from build123d import *

# Parameters (mm, degrees)
F0_R     = 60.325
F0_R_2   = 1.5875
F1_DEPTH = 3.175


with BuildPart() as f1:
    # F0 (on Front) → F1 (new body)
    with BuildSketch(Plane.XZ):
        Circle(F0_R)
        with BuildLine():
            ThreePointArc((-18.181951, -44.017693), (-39.585705, -26.478531), (-47.625, 0))
            Line((-47.625, 0), (-8.89, 0))
            ThreePointArc((-8.89, 0), (-7.82019, -4.228088), (-4.868239, -7.438571))
            Line((-4.868239, -7.438571), (-18.181951, -44.017693))
        make_face(mode=Mode.SUBTRACT)
        with BuildLine():
            ThreePointArc((0, -8.89), (4.228088, -7.82019), (7.438571, -4.868239))
            Line((7.438571, -4.868239), (44.017693, -18.181951))
            ThreePointArc((44.017693, -18.181951), (26.478531, -39.585705), (0, -47.625))
            Line((0, -47.625), (0, -8.89))
        make_face(mode=Mode.SUBTRACT)
        with BuildLine():
            Line((0, 47.625), (0, 8.89))
            ThreePointArc((0, 8.89), (-4.343939, 7.756436), (-7.580086, 4.644825))
            Line((-7.580086, 4.644825), (-44.11575, 17.94272))
            ThreePointArc((-44.11575, 17.94272), (-26.585885, 39.513685), (0, 47.625))
        make_face(mode=Mode.SUBTRACT)
        Circle(F0_R_2, mode=Mode.SUBTRACT)
        with BuildLine():
            ThreePointArc((8.89, 0), (7.82019, 4.228088), (4.868239, 7.438571))
            Line((4.868239, 7.438571), (18.181951, 44.017693))
            ThreePointArc((18.181951, 44.017693), (39.585705, 26.478531), (47.625, 0))
            Line((47.625, 0), (8.89, 0))
        make_face(mode=Mode.SUBTRACT)
    extrude(amount=F1_DEPTH)


solid = f1.part
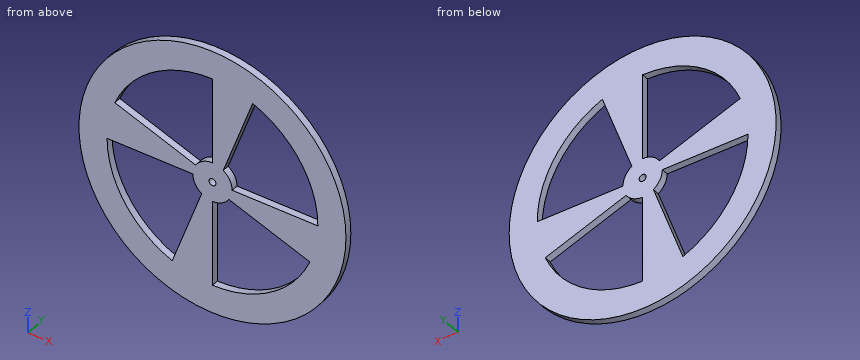
Here's how the part is built. I have some questions about the finished solid (model axes, mm). Coordinates: 2 decimals unless noted, no trailing zeros. Order: outer loops, then holes, each group sorted by start corner. A loop starts at its lowest first (then second) coordinate and runs counter-clockwise, first axis right, second up. Notation, with made-up numbers: (52.25, 26) -> (93.25, 26) arc R32 cw to (93.25, 63) -> close; hole circle Ø6 at (67.5, 63). An arc over 180 degrees is marked (long way). Answer in a Markdown table with one row per item.
(1) Please list where these lines run through material, in increasing order: probe 1 along X at (y, z) = (-2.65, 20); probe 2 along X at (y, z) = (-1.45, -23.5); probe 3 along Z at (x, y) = (-37, -2.25).
Answer key:
| item | result |
|---|---|
| probe 1 | -56.91 to -43.22, 0 to 9.44, 43.22 to 56.91 |
| probe 2 | -55.56 to -41.42, -10.71 to 0, 41.42 to 55.56 |
| probe 3 | -47.65 to -29.99, 0 to 15.35, 29.99 to 47.65 |
(2) I want a section at B-B on x = -42. List the corners of the cut face in (y, z) for me (3 decimals).
Answer key:
| item | result |
|---|---|
| outline | (-3.175, -43.302) -> (0, -43.302) -> (0, -22.453) -> (-3.175, -22.453) -> close; (-3.175, 0) -> (0, 0) -> (0, 17.173) -> (-3.175, 17.173) -> close; (-3.175, 22.453) -> (0, 22.453) -> (0, 43.302) -> (-3.175, 43.302) -> close |
(3) I want a section at C-C on z = -16. List the corners of the cut face in (x, y) for me (3 decimals), then the cut area to 3 significant figures.
Answer key:
| item | result |
|---|---|
| outline | (-58.164, -3.175) -> (-44.857, -3.175) -> (-44.857, 0) -> (-58.164, 0) -> close; (-7.984, -3.175) -> (0, -3.175) -> (0, 0) -> (-7.984, 0) -> close; (38.023, -3.175) -> (58.164, -3.175) -> (58.164, 0) -> (38.023, 0) -> close |
| area | 132 mm^2 |
(4) I want a section at A-A on y = -1.55. Count the separate pieces of the cut face and the enclosed holes in it, then the cut area to 3 significant figures.
Answer key:
| item | result |
|---|---|
| separate pieces | 1 |
| enclosed holes | 5 |
| area | 6,380 mm^2 |
(5) Will these pins go through, and if not, where does the flat tip stop? pin 1 Ø1 at (x, y) = (-31, -2) entering from -Z; pin 2 Ø1 at (y, z) = (-2, 33) entering from +X; pin 3 Ø1.6 at (y, z) = (-1.5, -37) entering from +X; pin 4 Ø3 at (x, z) = (0, 0) entering from -Y.
Answer key:
| item | result |
|---|---|
| pin 1 | z = -52.05 |
| pin 2 | x = 50.82 |
| pin 3 | x = 48.26 |
| pin 4 | through |
